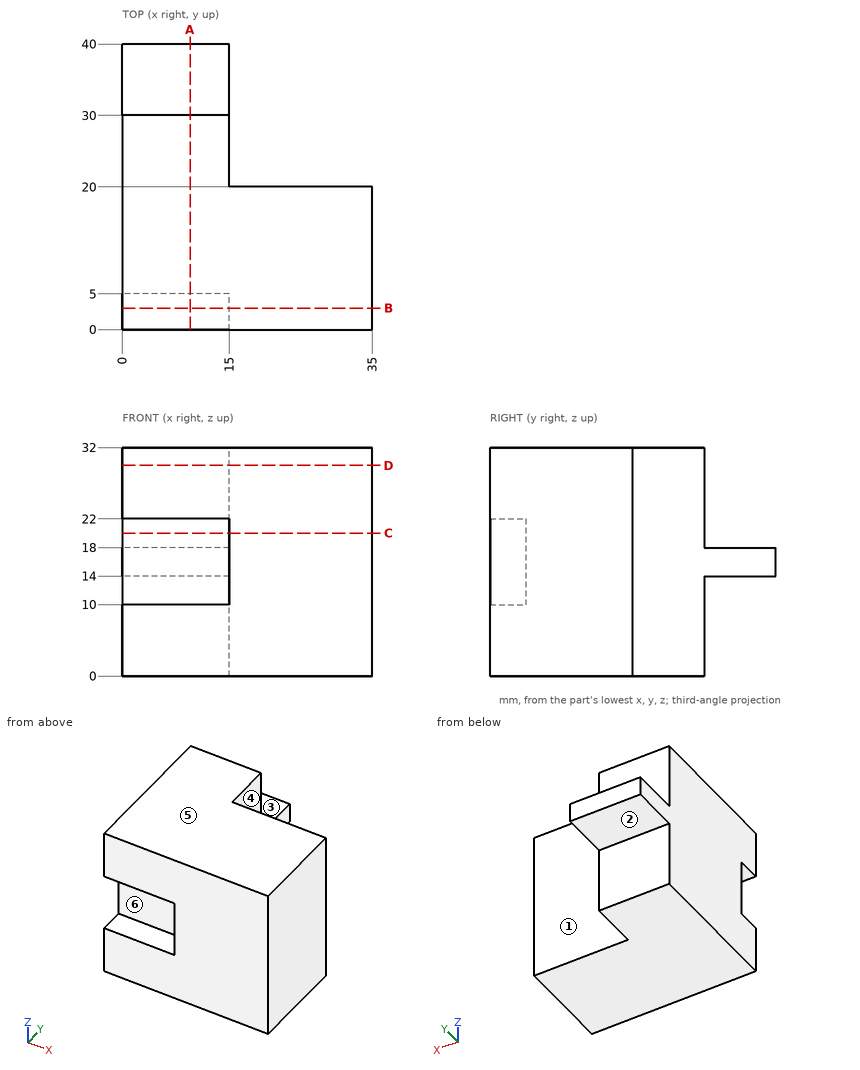
Input: dimensioned drawing with shaded views. Units: mm. Origin: part minimum x, y, z. A direction names the side the tool comes from. Coordinates: 2 decimals unless noted, no trailing zeros. Write each loop counter-clockwise with the first axis right and the second up, starting at its lowest first coordinate (ties: lowest second). Pieces come first, ordered by that corner, then holes. Notation, with made-up numbers: (-22.5, -3.75) -> (21.5, -3.75) arc R10 ccw to (21.5, 7.25) -> close; hole circle Ø11 at (-33.75, -0.5). An arc over 180 degrees is marked (long way). Return JSON: item names as keys, results as strings. Group by question number.
1) Section query A-A, the plane x = 9.5. Return loops of the section in (y, z).
2) Section query C-C, the plane z = 20. Return loops of the section in (x, y).
3) Section query D-D, the plane z = 29.5. Return loops of the section in (x, y), plus the area to 3 significant figures.
4) Contact query for flat-ended pins moving along their axis: P1, Ø12, axis at x = 17.5, z = 6.5, coming from the +Y side; P2, Ø2, axis at x = 26.5, z = 20, coming from the +Y side; P3, Ø3.5, axis at x = 9.5, z = 13.5, coming from the -Y side. Output: stop coordinate, or through.
5) Ray query, line 1 along Y through (x, z) = (9, 20.5); line 2 along Z through (x, y) = (6.5, 36); line 3 along X through (y, z) = (26, 2). Return the intervals inside material, ascending.
6) Mould query, pull axis Z, two halves, no side actions, for the marked faces 4, 5 and 6. Classes: +Z half, -Z half, draft (parallel to the pull), parting line (faces both ways), or undercut.
7) Set-up query: the marked faces 1, 2 and 3. Return all of +Z, -Z, +X, -X, +Y, -Y with unobstructed straight access to the full face (end or side cutting, diameter ignored); none if empty.
8) Section query B-B, the plane y = 3. Return loops of the section in (x, z), plus the area to 3 significant figures.
From the geometry:
{
 "1": {"outline": "(0, 0) -> (30, 0) -> (30, 14) -> (40, 14) -> (40, 18) -> (30, 18) -> (30, 32) -> (0, 32) -> (0, 22) -> (5, 22) -> (5, 10) -> (0, 10) -> close"},
 "2": {"outline": "(0, 5) -> (15, 5) -> (15, 0) -> (35, 0) -> (35, 20) -> (15, 20) -> (15, 30) -> (0, 30) -> close"},
 "3": {"outline": "(0, 0) -> (35, 0) -> (35, 20) -> (15, 20) -> (15, 30) -> (0, 30) -> close", "area": "850 mm²"},
 "4": {"P1": "y = 30", "P2": "y = 20", "P3": "y = 5"},
 "5": {"line 1": "5 to 30", "line 2": "14 to 18", "line 3": "0 to 15"},
 "6": {"face 4": "draft", "face 5": "+Z half", "face 6": "undercut"},
 "7": {"face 1": "+Z, -Z, +X, +Y", "face 2": "-Z, +X, -X, +Y", "face 3": "+Z, +X, -X, +Y"},
 "8": {"outline": "(0, 0) -> (35, 0) -> (35, 32) -> (0, 32) -> (0, 22) -> (15, 22) -> (15, 10) -> (0, 10) -> close", "area": "940 mm²"}
}
